Verification items for the finished model (mm, model axes). Face numbers are marked on the shaded views. A direction names the side the tool comes from. Coordinates: 2 decimals unless noted, no trailing zeros. Loops run counter-clockwise (first coordinate to the right, second up) from the corner with the lowest first, then second, coordinate; pieces in that order, holes last. Notation, with made-up numbers: (11.5, 31) - (68.5, 31) arc R29 cw to (68.5, 59) - close; hole circle Ø9 at (60.5, -39). An arc over 180 degrees is marked (long way). One line per item, written item: value. Start each with the question number.
(1) Draft check along Z on the marked faces 3, 4 and 5. Enter one of: +Z half, -Z half, draft (parallel to the pull), parting line (faces both ways), or undercut.
(2) Section check B-B (y = 22.5). Record the boundary of the cut face in (x, z).
(3) Set-up check for the marked faces 1 and 2: record each of +Z, -Z, +X, -X, +Y, -Y from which the full face is reachable in a straight line by a thin tool's end or side.
(4) Section check C-C (x = 7.5). Count the separate pieces of the cut face and the enclosed holes in it, plus the area to 3 significant figures.
(5) Section check A-A (z = 11.5). Record the boundary of the cut face in (x, y).
(6) Gauge pin test, flat ends, axial feed: P1, Ø3, axis at x = 7.5, y = 58, coming from the +Z side (3 decimals); P2, Ø4, axis at x = 13, y = 63.5, coming from the -Z side. Record the tip position at first contact, or that the pin passes through.
(7) Thickness scan on probe 1 along Y at (x, z) = (7.5, 0.85); probe 2 along X at (y, z) = (68, 11.25); probe 3 along X at (y, z) = (108.5, 14.3). Record the ranges inside material, lowest first. Write a range as [from, to].
Autodesk Inventor part; units mm, degrees
ref_plane "YZ Plane" through (0, 0, 0) normal (1, 0, 0) x (0, 1, 0)
ref_plane "XZ Plane" through (0, 0, 0) normal (0, 1, 0) x (-1, 0, 0)
ref_plane "XY Plane" through (0, 0, 0) normal (0, 0, 1) x (1, 0, 0)
sketch "スケッチ1" plane through (0, 0, 0) normal (0, 1, 0) x (-1, 0, 0)
  line L0 (0, 0) -> (-15, 0)
  line L1 (-15, 0) -> (-15, 15)
  line L2 (-15, 15) -> (0, 15)
  line L3 (0, 15) -> (0, 0)
  line L4 (-1.2, 13.8) -> (-13.8, 13.8)
  line L5 (-13.8, 13.8) -> (-13.8, 1.2)
  line L6 (-13.8, 1.2) -> (-1.2, 1.2)
  line L7 (-1.2, 1.2) -> (-1.2, 13.8)
  dimension "d0" = 15
  dimension "d1" = 15
  dimension "d2" = 1.2
  dimension "d3" = 1.2
  dimension "d4" = 1.2
  dimension "d5" = 1.2
extrude "押し出し1" add sketch "スケッチ1" along normal blind 116
sketch "スケッチ2" plane through (0, 0, 15) normal (0, 0, 1) x (1, 0, 0)
  line L0 (0, 116) -> (15, 116)
  line L1 (0, 0) -> (15, 0)
  line L2 (15, 0) -> (15, 116)
  point P0 (7.5, 108.5)
  point P1 (7.5, 7.5)
  dimension "d8" = 7.5
  dimension "d9" = 7.5
  dimension "d10" = 7.5
  dimension "d11" = 7.5
hole "穴1" at (7.5, 108.5, 15) at (7.5, 7.5, 15) direction (0, 0, -1) diameter 3 end through all
sketch "スケッチ3" plane through (15, 0, 15) normal (1, 0, 0) x (0, 0, -1)
  line L0 (0, 0) -> (15, 0)
  line L1 (0, 0) -> (0, 116)
  line L2 (0, 116) -> (15, 116)
  point P0 (7.5, 22.5)
  point P1 (7.5, 93.5)
  dimension "d19" = 22.5
  dimension "d20" = 7.5
  dimension "d21" = 7.5
  dimension "d22" = 22.5
hole "穴2" at (15, 22.5, 7.5) at (15, 93.5, 7.5) direction (-1, 0, 0) diameter 3 end through all
sketch "スケッチ4" plane through (15, 0, 0) normal (0, 0, -1) x (-1, 0, 0)
  line L0 (0, 116) -> (15, 116)
  line L1 (0, 0) -> (15, 0)
  line L2 (0, 0) -> (0, 116)
  point P0 (7.5, 58)
  dimension "d30" = 116
  dimension "d31" = 58
  dimension "d32" = 7.5
hole "穴3" at (7.5, 58, 0) direction (0, 0, 1) diameter 5 end through all
equation "\"d3\" = d2"
equation "\"d4\" = d2"
equation "\"d5\" = d2"
properties part number "ロボットベース15x15_4" material "アルミニウム 6061"
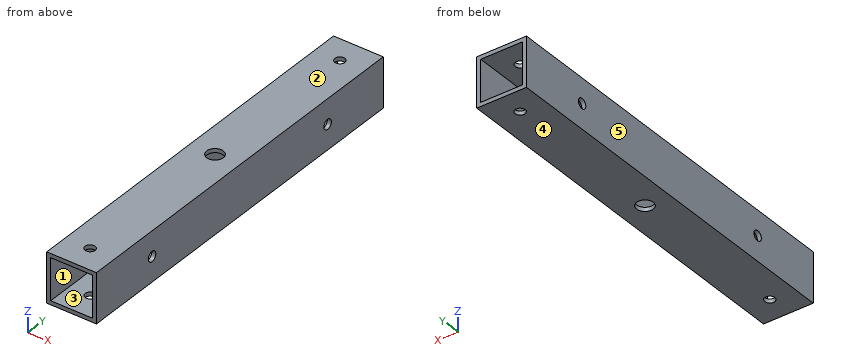
Responses:
1. face 3: undercut
1. face 4: -Z half
1. face 5: draft
2. outline: (0, 0) - (15, 0) - (15, 6) - (13.8, 6) - (13.8, 1.2) - (1.2, 1.2) - (1.2, 6) - (0, 6) - close; (0, 9) - (1.2, 9) - (1.2, 13.8) - (13.8, 13.8) - (13.8, 9) - (15, 9) - (15, 15) - (0, 15) - close
3. face 1: +Y, -Y
3. face 2: +Z, +X, -X, +Y, -Y
4. separate pieces: 8
4. enclosed holes: 0
4. area: 252 mm²
5. outline: (0, 0) - (1.2, 0) - (1.2, 116) - (0, 116) - close; (13.8, 0) - (15, 0) - (15, 116) - (13.8, 116) - close
6. P1: passes through
6. P2: stops at z = 0
7. probe 1: y = [0, 6], [9, 55.5], [60.5, 107], [110, 116]
7. probe 2: x = [0, 1.2], [13.8, 15]
7. probe 3: x = [0, 6], [9, 15]
